Input: dimensioned drawing with shaded views. Units: mm. Origin: part minimum x, y, z. Round coordinates to 2 decimals unless told otherwise and drop trailing zeros. Write each loop counter-clockwise with the first axis right and the second up, starting at its lowest first coordinate (ties: lowest second). Pieces come first, ordered by that corner, then holes. Notation, with made-up numbers: M 21,25 L 34,25 A10 ccw 34,43 Z; hole C -30.5,69 d11. An arc over 180 degrees is marked long. Put each result on its own line as item: value. Start each with the question number.
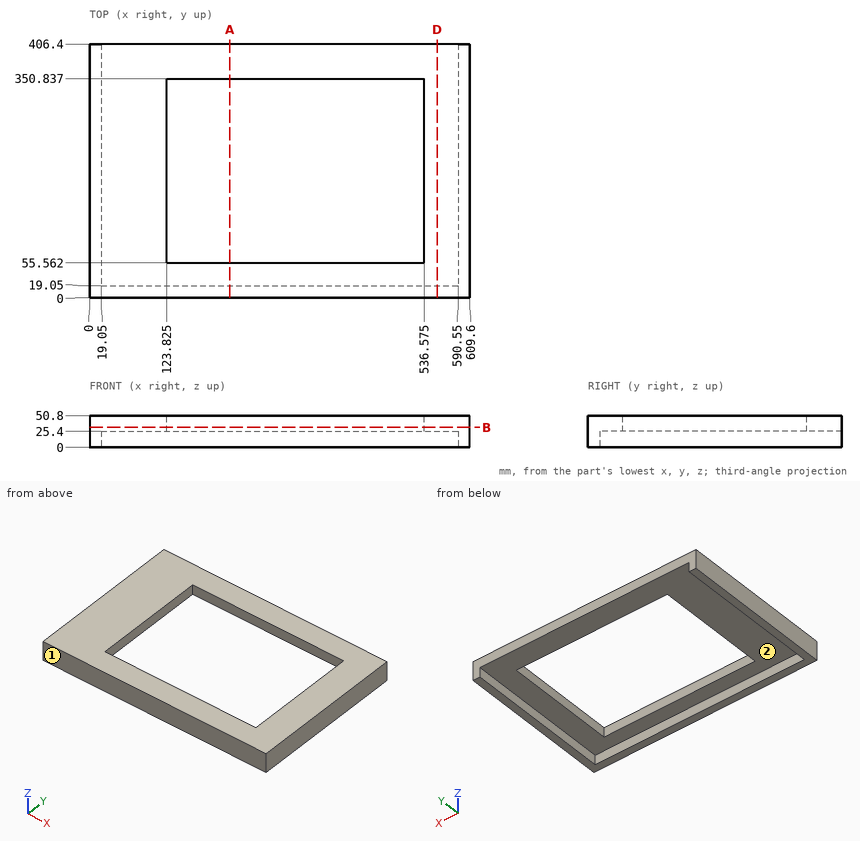
1) Section A-A, the plane x = 225. Output: boundary loops of the cut face in (y, z).
2) First-contact query: pin 1 (12.5 mm diameter, centred on x = 282.5, z = 14, fed in from +Y). Flat tip, straight axial feed; report the tip coordinate or a pass-through.
3) Section B-B, the plane z = 32. Output: boundary loops of the cut face in (x, y) (1 decimal).
4) Draft query along X for the marked faces 1 and 2. Return one class per face: +X half, -X half, draft (parallel to the pull), parting line (faces both ways), or undercut.
5) Ray query, probe 1 along X at (y, z) = (36, 7); probe 2 along X at (y, z) = (148.5, 46.5) (1 decimal); probe 3 along Y at (x, z) = (469.5, 41.5). Return the intervals inside material, ascending.
6) Section D-D, the plane x = 557. Output: boundary loops of the cut face in (y, z).
Solved:
1. outline: M 0,0 L 19.05,0 L 19.05,25.4 L 55.56,25.4 L 55.56,50.8 L 0,50.8 Z; M 350.84,25.4 L 406.4,25.4 L 406.4,50.8 L 350.84,50.8 Z
2. pin 1: stops at y = 19.05
3. outline: M 0,0 L 609.6,0 L 609.6,406.4 L 0,406.4 Z; hole M 123.8,55.6 L 536.6,55.6 L 536.6,350.8 L 123.8,350.8 Z
4. face 1: draft
4. face 2: undercut
5. probe 1: x = 0 to 19.05, 590.55 to 609.6
5. probe 2: x = 0 to 123.8, 536.6 to 609.6
5. probe 3: y = 0 to 55.56, 350.84 to 406.4
6. outline: M 0,0 L 19.05,0 L 19.05,25.4 L 406.4,25.4 L 406.4,50.8 L 0,50.8 Z
